from build123d import *

# Parameters (mm, degrees)
BOSS_EXTRU_1_DEPTH                        = 13.5
TROU_POUR_TARAUDAGE_POUR_TROU_TARAUD_M3_D = 2.5


with BuildPart() as part:
    # Esquisse1 → Boss.-Extru.1 (new body)
    with BuildSketch(Plane.XY):
        with BuildLine():
            Line((-3, 0), (3, 0))
            Line((3, 0), (3, -0.7))
            Line((3, -0.7), (4.05, -0.7))
            Line((4.05, -0.7), (4.05, -1.5))
            ThreePointArc((4.05, -1.5), (0, -4.5), (-4.05, -1.5))
            Line((-4.05, -1.5), (-4.05, -0.7))
            Line((-4.05, -0.7), (-3, -0.7))
            Line((-3, -0.7), (-3, 0))
        make_face()
    extrude(amount=BOSS_EXTRU_1_DEPTH)

    # Trou pour taraudage pour trou taraudé M31 (through all)
    with Locations(Plane(origin=(0, 0, 0), x_dir=(1, 0, 0), z_dir=(0, 1, 0))):
        with Locations((0, -9.5)):
            Hole(TROU_POUR_TARAUDAGE_POUR_TROU_TARAUD_M3_D / 2)

    # Esquisse4 → Révolution1 (revolve)
    with BuildSketch(Plane(origin=(0, 0, 0), x_dir=(0, 0, -1), z_dir=(1, 0, 0))):
        with BuildLine():
            Line((-3, -3.3), (-3, -5.3))
            ThreePointArc((-3, -5.3), (-2, -4.3), (-3, -3.3))
        make_face()
    revolve(axis=Axis((0, -3.3, 3), (0, -1, 0)))


solid = part.part
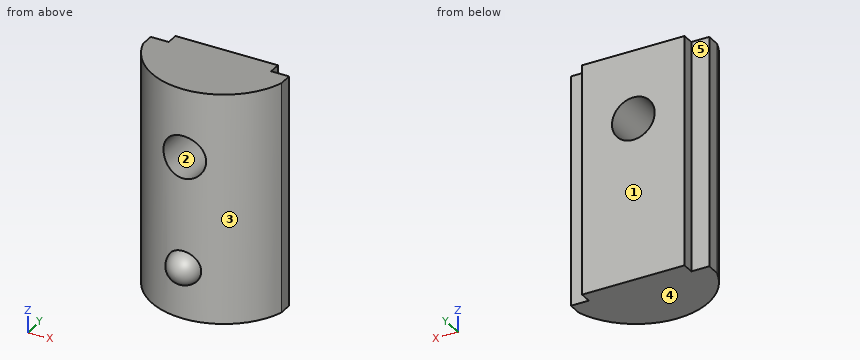
Build history of the part. All positions in model axes, mm. Face numbers are marked on the shaded views. A direction names the side the tool comes from. Round coordinates to 2 decimals unless told otherwise and drop trailing zeros. Write each loop counter-clockwise with the first axis right and the second up, starting at its lowest first coordinate (ties: lowest second). Pieces come first, ordered by that corner, then holes. Notation, with made-up numbers: (14.5, -35) - (54.5, -35) arc R31 ccw to (54.5, 3) - close; hole circle Ø11 at (-15, -12.5). An arc over 180 degrees is marked (long way). Use CSV: the item, a comma, the result in double quotes.
(1) Wall check: line 1 (Z direction, x = 0, y = -2.45); line 2 (X direction, y = -0.95, z = 9.5); line 3 (X direction, y = -1.9, z = 9.5). Give the ranges that are in metal, low to high.
Response:
line 1,"0 to 8.25, 10.75 to 13.5"
line 2,"-4.05 to -1.25, 1.25 to 4.05"
line 3,"-3.91 to -1.25, 1.25 to 3.91"
(2) Pin check, flat tips, straight feed: P1, Ø0.8, axis at x = 4, z = 8.5, coming from the +Y side; P2, Ø2, axis at x = -0.5, y = -2, coming from the -Z side; P3, Ø3, axis at x = -2, z = 2, coming from the -Y side; P4, Ø1, axis at x = 2.5, z = 2.5, coming from the -Y side. Stop position of each tip, or through.
Response:
P1,"y = -0.7"
P2,"z = 0"
P3,"y = -4.98"
P4,"y = -4"
(3) Band-saw the part on A-A (x = -0.25). Write the cut outline in (y, z).
Response:
outline,"(-4.49, 0) - (0, 0) - (0, 8.28) - (-4.49, 8.28) - (-4.49, 3.95) arc R0.97 ccw to (-4.49, 2.05) - close; (-4.49, 10.72) - (0, 10.72) - (0, 13.5) - (-4.49, 13.5) - close"
(4) Band-saw the part on B-B (z = 8.5). Write the cut outline in (x, y).
Response:
outline,"(-4.05, -1.5) arc R4.23 ccw to (-0.75, -4.43) - (-0.75, 0) - (-3, 0) - (-3, -0.7) - (-4.05, -0.7) - close; (0.75, -4.43) arc R4.23 ccw to (4.05, -1.5) - (4.05, -0.7) - (3, -0.7) - (3, 0) - (0.75, 0) - close"
(5) Mould opens along X. For the marked faces 1, 2 and 3 say: pulls with the +X half, pulls with the -X half, needs draft (parallel to the pull), parting line crosses it, or undercut.
Response:
face 1,"needs draft"
face 2,"undercut"
face 3,"parting line crosses it"
(6) Band-saw the part on C-C (y = -0.35). Write the cut outline in (x, z), plus the area to 3 significant figures.
Response:
outline,"(-3, 0) - (3, 0) - (3, 13.5) - (-3, 13.5) - close; hole circle Ø2.5 at (0, 9.5)"
area,"76.1 mm²"
(7) 3-axis set-ups, long thin cutter, end or side, ignore diameter. For the marked faces 4 and 5: which of +Z, -Z, +X, -X, +Y, -Y reach the whole face in a straight line?
Response:
face 4,"-Z, +X, -X, +Y, -Y"
face 5,"+Z, -Z, -X, +Y"
(8) Band-saw the part on D-D (y = -3). Write the cut outline in (x, z).
Response:
outline,"(-3.23, 0) - (3.23, 0) - (3.23, 13.5) - (-3.23, 13.5) - close; hole circle Ø2.5 at (0, 9.5)"
